Study the drawing (mm; zero at the part's minimum x, y, z) and answer. A direction names the side the tool comes from. Coordinates: 2 decimals unless noted, no trailing zeros. Order: outer loops, then holes, each group sorted by start corner. A loop starts at its lowest first (then second) coordinate and runs counter-clockwise, first axis right, second up.
1. The part is cut by section C-C, the plane x = 40. Give the vertices of the cut face in (y, z), then the cut area to 3 significant figures.
2. The part is cut by section A-A, the plane z = 2. Give the vertices of the cut face in (x, y).
3. Flat-ended cylindrical pins translate along their axes: pin 1 Ø8 at (y, z) = (48.5, 12.5) entering from +X; pin 2 Ø1.8 at (y, z) = (52, 10.5) entering from +X; pin 3 Ø12 at (x, z) = (28.5, 29) entering from -Y. Find the tip coordinate at first contact, or state that the pin passes through.
4. A tool of negligible diameter and unlimited length cuts with its end or side. For the marked faces 1, 2, 3, 4 and 5, from which of +Z, -Z, +X, -X, +Y, -Y can it reach the whole face along a straight path? Write none if from no direction.
5. Determine the mould class of the marked faces 6, 7, 8 and 9 for opening direction X: +X half, -X half, draft (parallel to the pull), parting line (faces both ways), or undercut.
6. The part is cut by section D-D, the plane z = 18. Give the vertices of the cut face in (x, y).
7. Find the intervals of material crossed by probe 1 along X at (y, z) = (16, 29); probe 2 along Z at (x, y) = (29.5, 29.5); probe 3 along Y at (x, z) = (19.5, 32), in increasing order.
8. The part is cut by section B-B, the plane y = 50. Give the vertices of the cut face in (x, z).
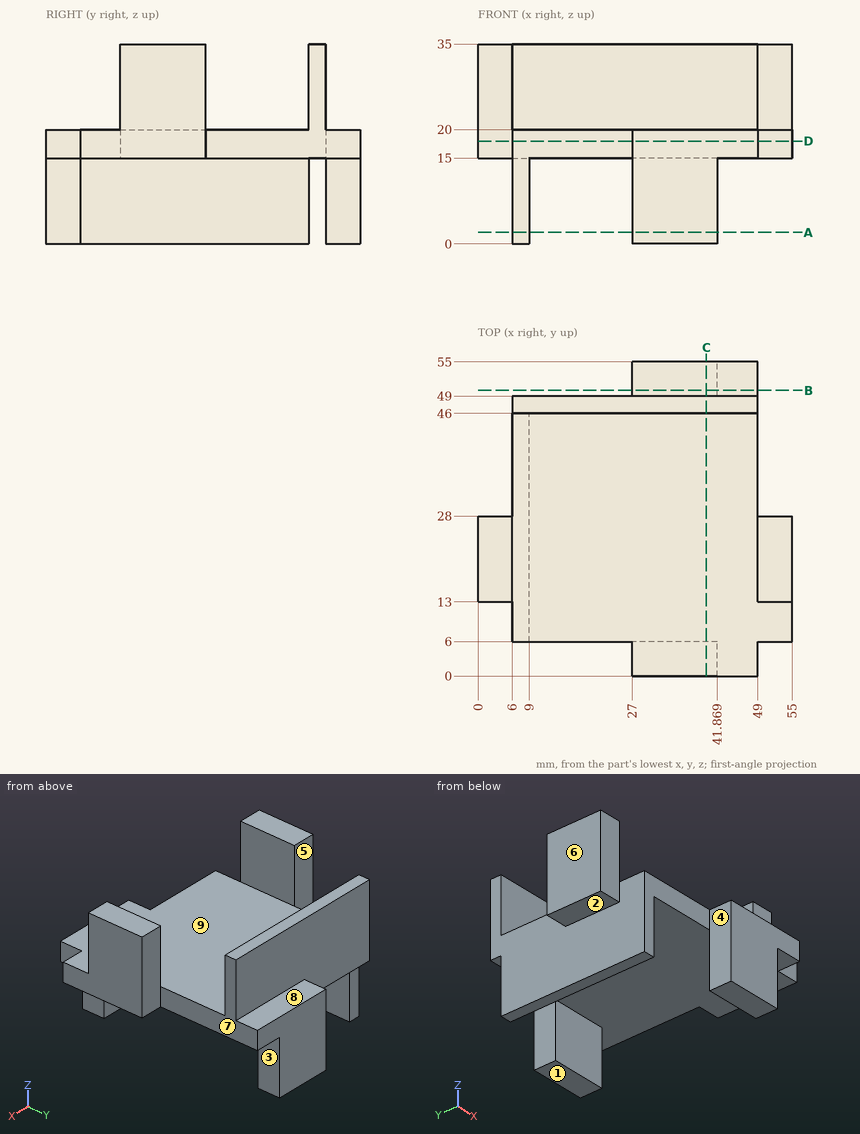
Geometry says:
1. outline: (0, 0) - (6, 0) - (6, 15) - (49, 15) - (49, 0) - (55, 0) - (55, 20) - (49, 20) - (49, 35) - (46, 35) - (46, 20) - (0, 20) - close
1. area: 500 mm2
2. outline: (6, 6) - (9, 6) - (9, 46) - (6, 46) - close; (27, 0) - (41.87, 0) - (41.87, 6) - (27, 6) - close; (27, 49) - (41.87, 49) - (41.87, 55) - (27, 55) - close
3. pin 1: stops at x = 49
3. pin 2: stops at x = 41.87
3. pin 3: stops at y = 46
4. face 1: -Z, +X, -X, +Y, -Y
4. face 2: -Z, -X, +Y, -Y
4. face 3: -Z, +X, +Y, -Y
4. face 4: +Z, -Z, -X, -Y
4. face 5: +Z, -Z, -X, +Y
5. face 6: -X half
5. face 7: +X half
5. face 8: draft
5. face 9: undercut
6. outline: (0, 13) - (6, 13) - (6, 6) - (27, 6) - (27, 0) - (49, 0) - (49, 6) - (55, 6) - (55, 28) - (49, 28) - (49, 55) - (27, 55) - (27, 49) - (6, 49) - (6, 28) - (0, 28) - close
7. probe 1: x = 0 to 6, 49 to 55
7. probe 2: z = 15 to 20
7. probe 3: y = 46 to 49
8. outline: (27, 0) - (41.87, 0) - (41.87, 15) - (49, 15) - (49, 20) - (27, 20) - close
